Build history of the part. All positions in model axes, mm. Round coordinates to 2 decimals unless told otherwise and drop trailing zeros. Write each loop counter-clockwise with the first axis right and the second up, starting at its lowest first coordinate (ties: lowest second). Pieces come first, ordered by that corner, then holes.
1) Flat gauge pin, fed straight in: pin 1 (5 mm diameter, centred on x = -37, z = -55.5, fed in from -Y). Where does the tip first touch, or does it go through?
2) Saw through at C-C (z = -16). Write the cut outline in (x, y).
3) Wall check: probe 1 along X at (y, z) = (1.4, -13.5); probe 2 along Z at (x, y) = (-22, 0.45). Give the ranges that are in metal, low to high.
4) Saw through at B-B (y = 1.7). Write the cut outline in (x, z).
5) Saw through at A-A (x = 9.5). Write the cut outline in (y, z), plus the area to 3 significant figures.
from build123d import *

# Parameters (mm, degrees)
SKETCH1_W           = 230
SKETCH1_H           = 230
BOSS_EXTRUDE1_DEPTH = 3


with BuildPart() as part:
    # Sketch1 → Boss-Extrude1 (new body)
    with BuildSketch(Plane(origin=(0, 0, 0), x_dir=(1, 0, 0), z_dir=(0, 1, 0))):
        Rectangle(SKETCH1_W, SKETCH1_H)
        with BuildLine():
            Line((-20, -35), (20, -35))
            ThreePointArc((20, -35), (30.606601718, -30.606601718), (35, -20))
            Line((35, -20), (35, 20))
            ThreePointArc((35, 20), (30.606601718, 30.606601718), (20, 35))
            Line((20, 35), (-20, 35))
            ThreePointArc((-20, 35), (-30.606601718, 30.606601718), (-35, 20))
            Line((-35, 20), (-35, -20))
            ThreePointArc((-35, -20), (-30.606601718, -30.606601718), (-20, -35))
        make_face(mode=Mode.SUBTRACT)
    extrude(amount=BOSS_EXTRUDE1_DEPTH)


solid = part.part
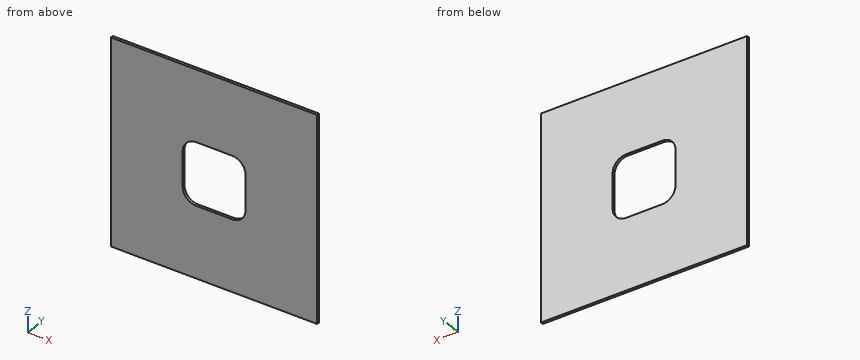
Evaluation:
1. pin 1: stops at y = 0
2. outline: (-115, 0) - (-35, 0) - (-35, 3) - (-115, 3) - close; (35, 0) - (115, 0) - (115, 3) - (35, 3) - close
3. probe 1: x = -115 to -35, 35 to 115
3. probe 2: z = -115 to -34.87, 34.87 to 115
4. outline: (-115, -115) - (115, -115) - (115, 115) - (-115, 115) - close; hole (-35, -20) arc R15 ccw to (-20, -35) - (20, -35) arc R15 ccw to (35, -20) - (35, 20) arc R15 ccw to (20, 35) - (-20, 35) arc R15 ccw to (-35, 20) - close
5. outline: (0, -115) - (3, -115) - (3, -35) - (0, -35) - close; (0, 35) - (3, 35) - (3, 115) - (0, 115) - close
5. area: 480 mm2
